Read the model definition and answer for the solid it produces. Units are mm, in the model's axes. A direction names the side the tool comes from. Round coordinates to 2 decimals unless told otherwise and drop trailing zeros. Order: outer loops, then holes, each group sorted by start corner. A loop starts at its lowest first (then second) coordinate and runs counter-clockwise, first axis right, second up. Notation, with made-up numbers: M -34,54 L -19,54 A14 cw -19,73 Z; hole C 67,-32 d11. An arc over 180 degrees is marked long. Answer as CSV lines item,"result".
```python
from build123d import *

# Parameters (mm, degrees)
BOSS_EXTRUDE1_DEPTH = 5
SKETCH2_R           = 4
BOSS_EXTRUDE2_DEPTH = 35


with BuildPart() as part:
    # Sketch1 → Boss-Extrude1 (new body)
    with BuildSketch(Plane(origin=(0, 0, 0), x_dir=(1, 0, 0), z_dir=(0, 1, 0))):
        Polygon((3.970106574, -5.677874056), (6.902236459, 0.599276121), (2.932129885, 6.277150177), (-3.970106574, 5.677874056), (-6.902236459, -0.599276121), (-2.932129885, -6.277150177), align=None)
    extrude(amount=BOSS_EXTRUDE1_DEPTH)

    # Sketch2 → Boss-Extrude2 (add)
    with BuildSketch(Plane(origin=(0, 5, 0), x_dir=(1, 0, 0), z_dir=(0, 1, 0))):
        with Locations(Location((0, 0, 0), (0, 0, 270))):
            Circle(SKETCH2_R)
    extrude(amount=BOSS_EXTRUDE2_DEPTH)


solid = part.part
```
Item 1: Find the intervals of material crossed by probe 1 along Z at (x, y) = (-0.25, 37.5); probe 2 along Y at (x, z) = (-3.25, -4), in increasing order. Write a range as [from, to].
Ans:
probe 1,"[-3.99, 3.99]"
probe 2,"[0, 5]"
Item 2: A cutting plane is placed at B-B, the plane x = -2. Determine the outline of the cut face in (y, z), and give its area (3 significant figures).
Ans:
outline,"M 0,-5.85 L 5,-5.85 L 5,-3.46 L 40,-3.46 L 40,3.46 L 5,3.46 L 5,6.2 L 0,6.2 Z"
area,"303 mm2"
Item 3: A cutting plane is placed at C-C, the plane y = 14. Determine the outline of the cut face in (x, z).
Ans:
outline,"C 0,0 d8"
Item 4: A cutting plane is placed at A-A, the plane z = 0. Determine the outline of the cut face in (x, y).
Ans:
outline,"M -6.62,0 L 6.62,0 L 6.62,5 L 4,5 L 4,40 L -4,40 L -4,5 L -6.62,5 Z"
Item 5: Flat-ended cylindrical pins translate along their axes: pin 1 (1.5 mm diameter, centred on y = 6, z = 5, fed in from +X); pin 2 (1.5 mm diameter, centred on x = -4.5, z = -3.5, fed in from +Y); pin 3 (1 mm diameter, centred on x = 3, y = 22, fed in from -Z); pin 4 (1.5 mm diameter, centred on y = 26, z = 2, fed in from -X). Find the tip coordinate at first contact, or state that the pin passes through.
Ans:
pin 1,"through"
pin 2,"y = 5"
pin 3,"z = -3.12"
pin 4,"x = -3.8"
Item 6: A tool of negligible diameter and unlimited length cuts with its end or side. For faces 1 (the face through (3, 5, 3)), 2 (the face through (-0.47, 2.46, -5.98)), from which of +Z, -Z, +X, -X, +Y, -Y can it reach the whole face along a straight path? Write none if from no direction.
Ans:
face 1,"+Y"
face 2,"-Z, -X, +Y, -Y"
Item 7: A cutting plane is placed at D-D, the plane x = -5.5. Determine the outline of the cut face in (y, z), and give its area (3 significant figures).
Ans:
outline,"M 0,-2.4 L 5,-2.4 L 5,2.6 L 0,2.6 Z"
area,"25.0 mm2"
